from build123d import *

# Parameters (mm, degrees)
CHAMFER1_SIZE                = 1
CHAMFER2_SIZE                = 0.5
M10_TAPPED_HOLE1_D           = 10
M10_TAPPED_HOLE1_CSINK_D     = 12
M10_TAPPED_HOLE1_CSINK_ANGLE = 90


with BuildPart() as part:
    # Sketch1 → Revolve1 (revolve)
    with BuildSketch(Plane.XY, mode=Mode.PRIVATE) as revolve1_sk:
        Polygon((0, 9.525), (-5, 9.525), (-5, 0), (20, 0), (20, 7.525), (0, 7.525), align=None)
    revolve(revolve1_sk.sketch.rotate(Axis((-15.231671031, 0, 0), (1, 0, 0)), 90), axis=Axis((-15.231671031, 0, 0), (1, 0, 0)))

    # Chamfer1
    chamfer1_edges = [part.edges().sort_by_distance(p)[0] for p in [
        (20, 0, -7.525),
        (-5, 0, -9.525),
    ]]
    chamfer(chamfer1_edges, length=CHAMFER1_SIZE)

    # Chamfer2
    chamfer2_edges = [part.edges().sort_by_distance(p)[0] for p in [
        (0, 0, -9.525),
    ]]
    chamfer(chamfer2_edges, length=CHAMFER2_SIZE)

    # M10 Tapped Hole1 (through all)
    with Locations(Plane.ZY.offset(5)):
        with Locations((0, 0)):
            CounterSinkHole(M10_TAPPED_HOLE1_D / 2, M10_TAPPED_HOLE1_CSINK_D / 2, counter_sink_angle=M10_TAPPED_HOLE1_CSINK_ANGLE)


solid = part.part
Build history of the part. All positions in model axes, mm. A direction names the side the tool comes from. Round coordinates to 2 decimals unless told otherwise and drop trailing zeros. Write each loop counter-clockwise with the first axis right and the second up, starting at its lowest first coordinate (ties: lowest second). Pieces come first, ordered by that corner, then holes. Notation, with made-up numbers: M 42.25,89 L 93.25,89 A27 ccw 93.25,128 Z; hole C 31.25,74 d11. An arc over 180 degrees is marked long. Answer as a JSON object with one key per item and string values. Group by question number.
(1) Mould opens along Z. For faces 1 (the cylindrical face through (8.17, -4.88, 1.08)), 2 (the flat face through (20, 5, -2)), 3 (the cylindrical face through (-2.27, 9.3, -2.06)) say: pulls with the +Z half, pulls with the -Z half, needs draft (parallel to the pull), parting line crosses it, or undercut.
(2) Cut at A-A (z = 0). Give the cut face in (x, y) (3 decimals).
(3) Which spindle directions (+Z, -Z, +X, -X, +Y, -Y) get a long thin tool onto all of the face, cutting with end or side? Do faces 4 (the flat face through (-5, 2, -6)), 5 (the flat face through (0, 6, 5)). Say none if no direction does.
(4) Flat gauge pins, fed straight in: pin 1 (2 mm diameter, centred on y = 3, z = -6, fed in from +X); pin 2 (1 mm diameter, centred on x = 2, y = 5, fed in from +Z); pin 3 (1 mm diameter, centred on x = 16.5, y = -1, fed in from -Z); pin 4 (4 mm diameter, centred on x = 13.5, z = -6.5, fed in from -Y). Where does each tip first touch, or does it go through?
(5) Cut at C-C (x = -1.25). Give the cut face in (y, z) (3 decimals), and give its area (3 significant figures).
(6) Cut at D-D (x = 3.25). Give the cut face in (y, z) (3 decimals), and give its area (3 significant figures).
(7) Drill centre lines: L1, parallel to Y at x = 5.75, z = 0.25; L2, parallel to X at y = 7.5, z = -1; L3, parallel to Z at x = 3.5, y = 1.75. Where is each one in solid material? Low to high.
Responses:
{
 "1": {"face 1": "undercut", "face 2": "needs draft", "face 3": "parting line crosses it"},
 "2": {"outline": "M -5,-8.525 L -4,-9.525 L -0.5,-9.525 L 0,-9.025 L 0,-7.525 L 19,-7.525 L 20,-6.525 L 20,-5 L -4,-5 L -5,-6 Z; M -5,6 L -4,5 L 20,5 L 20,6.525 L 19,7.525 L 0,7.525 L 0,9.025 L -0.5,9.525 L -4,9.525 L -5,8.525 Z"},
 "3": {"face 4": "+Z, -Z, -X, +Y, -Y", "face 5": "+X"},
 "4": {"pin 1": "stops at x = 20", "pin 2": "stops at z = 6.03", "pin 3": "stops at z = -7.51", "pin 4": "stops at y = -6.03"},
 "5": {"outline": "C 0,0 d19.05; hole C 0,0 d10", "area": "206 mm2"},
 "6": {"outline": "C 0,0 d15.05; hole C 0,0 d10", "area": "99.4 mm2"},
 "7": {"L1": "y = -7.52 to -4.99, 4.99 to 7.52", "L2": "x = -5 to 0", "L3": "z = -7.32 to -4.68, 4.68 to 7.32"}
}
